from build123d import *

# Parameters (mm, degrees)
F0_R      = 49.9014426293
F1_DEPTH  = 127
F2_R      = 37.9248906149
F3_DEPTH  = 152.4
F4_SIZE   = 5.08
F6_DEPTH  = 25.4
F9_W      = 24.138873443
F9_H      = 129.7791451216
F10_DEPTH = 50.8


# Not quite as in the source:
# - the program builds the solid bodies; features that only make, move or delete a surface that nothing else refers to are left out


with BuildPart() as f1:
    # F0 (on Front) → F1 (new body)
    with BuildSketch(Plane.XZ):
        Circle(F0_R)
    extrude(amount=F1_DEPTH)

    # F2 (on face) → F3 (join)
    with BuildSketch(Plane.XZ.offset(127)):
        Circle(F2_R)
    extrude(amount=F3_DEPTH)

    # F4
    f4_edges = [f1.edges().sort_by_distance(p)[0] for p in [
        (-49.901443, -127, 0),
        (-37.924891, -127, 0),
        (-37.924891, -279.4, 0),
        (-49.901443, 0, 0),
    ]]
    chamfer(f4_edges, length=F4_SIZE)

    # F5 (on face) → F6 (cut)
    with BuildSketch(Plane.XZ.offset(279.4)):
        Polygon((-13.8807385989, -29.7676323455), (18.8391565222, -26.9048884227), (32.7198951211, 2.8627439228), (13.8807385989, 29.7676323455), (-18.8391565222, 26.9048884227), (-32.7198951211, -2.8627439228), align=None)
    extrude(amount=-F6_DEPTH, mode=Mode.SUBTRACT)

    # F9 (on face) → F10 (cut)
    with BuildSketch(Plane(origin=(0, 0, 0), x_dir=(-1, 0, 0), z_dir=(0, 1, 0))):
        Rectangle(F9_W, F9_H)
    extrude(amount=-F10_DEPTH, mode=Mode.SUBTRACT)


solid = f1.part
Design review of the part built by this model. Coordinates are the model's own, in mm. A direction names the side the tool comes from. Round coordinates to 2 decimals unless told otherwise and drop trailing zeros. Order: outer loops, then holes, each group sorted by start corner. A loop starts at its lowest first (then second) coordinate and runs counter-clockwise, first axis right, second up. Notation, with made-up numbers: M 40.25,-27.75 L 69.25,-27.75 A26 ccw 69.25,4.25 Z; hole C 1,31 d1. An arc over 180 degrees is marked long. Answer as CSV lines item,"result". Start each with the question number.
1) Add section C-C (z = 0). Give the boundary of the cut face in (x, y), then the cut area to 3 significant figures.
2) The part is to be moulded in two halves that separate along Z. For faces 1 (the face through (27, -279.4, -13)), 2 (the face through (-45.06, -0.247, 0.837)), 3 (the face through (-25.68, -266.88, 12.23)), say which applies: +Z half, -Z half, draft (parallel to the pull), parting line (faces both ways), or undercut.
3) Add section D-D (y = -197). Give the boundary of the cut face in (x, z).
4) Wall thickness on line 1 along X through (y, z) = (-12, -12); line 2 along Z through (x, y) = (0, -242); line 3 along Y through (x, z) = (5.5, 11): over which ranges is each line inside the solid? List them lowest first. Write a range as [from, to].
5) Tool access review of faces 4 (the face through (0, -254, 0)), 5 (the face through (12.069, -25, -1)), 6 (the face through (45.06, -0.247, -0.837)): name each direction out of +Z, -Z, +X, -X, +Y, -Y from which nothing blocks a thin tool from reaching the whole face with its end or side.
6) Add section B-B (x = 0). Give the boundary of the cut face in (y, z).
7) Add section A-A (y = -40.5). Give the boundary of the cut face in (x, z), then the cut area to 3 significant figures.
8) For pin 1 Ø3 at (y, z) = (-152, -24.5) entering from -X; pin 2 Ø2 at (x, z) = (30, -37) entering from -Y; pin 3 Ø12 at (x, y) = (-2.5, -226.5) entering from +Z, all flat-tipped, find the tip position at first contact; note any pin that passes through.
Resolved:
1,outline,"M -49.9,-121.92 L -44.82,-127 L -43,-127 L -37.92,-132.08 L -37.92,-274.32 L -32.84,-279.4 L -31.38,-279.4 L -31.38,-254 L 31.38,-254 L 31.38,-279.4 L 32.84,-279.4 L 37.92,-274.32 L 37.92,-132.08 L 43,-127 L 44.82,-127 L 49.9,-121.92 L 49.9,-5.08 L 44.82,0 L 12.07,0 L 12.07,-50.8 L -12.07,-50.8 L -12.07,0 L -44.82,0 L -49.9,-5.08 Z"
1,area,"21,400 mm^2"
2,face 1,"draft"
2,face 2,"parting line"
2,face 3,"undercut"
3,outline,"C 0,0 d75.85"
4,line 1,"[-48.44, -12.07], [12.07, 48.44]"
4,line 2,"[-37.92, 37.92]"
4,line 3,"[-254, -50.8]"
5,face 4,"-Y"
5,face 5,"+Z, -Z, +Y"
5,face 6,"+X, +Y"
6,outline,"M -279.4,-32.84 L -274.32,-37.92 L -132.08,-37.92 L -127,-43 L -127,-44.82 L -121.92,-49.9 L -50.8,-49.9 L -50.8,49.9 L -121.92,49.9 L -127,44.82 L -127,43 L -132.08,37.92 L -274.32,37.92 L -279.4,32.84 L -279.4,28.55 L -254,28.55 L -254,-28.55 L -279.4,-28.55 Z"
7,outline,"M -12.07,-48.42 L -12.07,48.42 A49.9 ccw Z; M 12.07,-48.42 A49.9 ccw 12.07,48.42 Z"
7,area,"5,440 mm^2"
8,pin 1,"x = -30.15"
8,pin 2,"y = -125.19"
8,pin 3,"z = 37.92"
